from build123d import *

# Parameters (mm, degrees)
SKETCH_1_W      = 40
SKETCH_1_H      = 40
EXTRUDE_1_DEPTH = 20
CHAMFER_2_SIZE  = 2
SKETCH_2_R      = 5
EXTRUDE_3_DEPTH = 2
SKETCH_4_R      = 2.5
EXTRUDE_6_DEPTH = 3
CHAMFER_3_SIZE  = 2
FILLET_1_R      = 2


with BuildPart() as part:
    # 草图1 → 凸台-拉伸1 (new body)
    with BuildSketch(Plane.XY):
        with Locations((-8.736097926, 20.42824298)):
            Rectangle(SKETCH_1_W, SKETCH_1_H)
    extrude(amount=EXTRUDE_1_DEPTH)

    # 倒角2
    chamfer_2_edges = [part.edges().sort_by_distance(p)[0] for p in [
        (-8.736097926, 40.42824298, 20),
        (-8.736097926, 40.42824298, 0),
        (-28.736097926, 40.42824298, 10),
        (11.263902074, 40.42824298, 10),
    ]]
    chamfer(chamfer_2_edges, length=CHAMFER_2_SIZE)

    # 草图2 → 凸台-拉伸3 (add)
    with BuildSketch(Plane(origin=(0, 0.42824298, 0), x_dir=(-1, 0, 0), z_dir=(0, -1, 0))):
        with Locations(Location((18.736097926, -10, 0), (0, 0, 270))):
            Circle(SKETCH_2_R)
    extrude(amount=EXTRUDE_3_DEPTH)

    # 草图4 → 凸台-拉伸6 (add)
    with BuildSketch(Plane.XZ.offset(1.57175702)):
        with Locations(Location((-18.736097926, 10, 0), (0, 0, 270))):
            Circle(SKETCH_4_R)
    extrude(amount=EXTRUDE_6_DEPTH)

    # 倒角3
    chamfer_3_edges = [part.edges().sort_by_distance(p)[0] for p in [
        (-8.736097926, 0.42824298, 20),
        (-8.736097926, 0.42824298, 0),
        (-28.736097926, 0.42824298, 10),
        (11.263902074, 0.42824298, 10),
    ]]
    chamfer(chamfer_3_edges, length=CHAMFER_3_SIZE)

    # 圆角1
    fillet_1_edges = [part.edges().sort_by_distance(p)[0] for p in [
        (11.263902074, 20.42824298, 0),
        (11.263902074, 20.42824298, 20),
        (-28.736097926, 20.42824298, 0),
        (-28.736097926, 20.42824298, 20),
    ]]
    fillet(fillet_1_edges, radius=FILLET_1_R)


solid = part.part
Model file for the job. Use its own axes, mm. A direction names the side the tool comes from. Round coordinates to 2 decimals unless told otherwise and drop trailing zeros. Loops run counter-clockwise (first coordinate to the right, second up) from the corner with the lowest first, then second, coordinate; pieces in that order, holes last. Notation, with made-up numbers: (67.25, -27.5) - (93.25, -27.5) arc R16 ccw to (93.25, -17.5) - close; hole circle Ø9 at (38, 83). An arc over 180 degrees is marked (long way). Write each question's results on one line, items separated by ' | '.
(1) Saw through at D-D, the plane x = -18. List the corners of the cut face in (y, z), then the cut area to 3 significant figures.
Answer below:
outline: (-4.57, 7.61) - (-1.57, 7.61) - (-1.57, 5.05) - (0.43, 5.05) - (0.43, 2) - (2.43, 0) - (38.43, 0) - (40.43, 2) - (40.43, 18) - (38.43, 20) - (2.43, 20) - (0.43, 18) - (0.43, 14.95) - (-1.57, 14.95) - (-1.57, 12.39) - (-4.57, 12.39) - close | area: 826 mm^2
(2) Pin check, flat tips, straight feed: pin 1 (6 mm diameter, centred on x = 7, z = 12, fed in from -Y); pin 2 (3 mm diameter, centred on x = -14, z = 7, fed in from -Y). Stop position of each tip, or through.
Answer below:
pin 1: stops at y = 0.43 | pin 2: stops at y = -1.57
(3) Wall check: L1, parallel to Y at x = -23, z = 3.5; L2, parallel to Y at x = -23, z = 9.5; L3, parallel to Z at x = -16.5, y = 0. Give the ranges that are in metal, low to high.
Answer below:
L1: y = 0.43 to 40.43 | L2: y = -1.57 to 40.43 | L3: z = 5.53 to 14.47
(4) Saw through at A-A, the plane x = -11.5. List the corners of the cut face in (y, z), then the cut area to 3 significant figures.
Answer below:
outline: (0.43, 2) - (2.43, 0) - (38.43, 0) - (40.43, 2) - (40.43, 18) - (38.43, 20) - (2.43, 20) - (0.43, 18) - close | area: 792 mm^2
(5) Saw through at C-C, the plane z = 6. List the corners of the cut face in (x, y), then the cut area to 3 significant figures.
Answer below:
outline: (-28.74, 2.43) - (-26.74, 0.43) - (-21.74, 0.43) - (-21.74, -1.57) - (-15.74, -1.57) - (-15.74, 0.43) - (9.26, 0.43) - (11.26, 2.43) - (11.26, 38.43) - (9.26, 40.43) - (-26.74, 40.43) - (-28.74, 38.43) - close | area: 1,600 mm^2
(6) 3-axis set-ups, long thin cutter, end or side, ignore diameter. For faces 1 (the flat face through (-16.6, -1.572, 12.2)), 2 (the flat face through (-27.72, 1.41, 9.87)): which of +Z, -Z, +X, -X, +Y, -Y reach the whole face in a straight line?
Answer below:
face 1: -Y | face 2: +Z, -Z, -X, -Y
(7) Saw through at B-B, the plane z = 10. List the corners of the cut face in (x, y), then the cut area to 3 significant figures.
Answer below:
outline: (-28.74, 2.43) - (-26.74, 0.43) - (-23.74, 0.43) - (-23.74, -1.57) - (-21.24, -1.57) - (-21.24, -4.57) - (-16.24, -4.57) - (-16.24, -1.57) - (-13.74, -1.57) - (-13.74, 0.43) - (9.26, 0.43) - (11.26, 2.43) - (11.26, 38.43) - (9.26, 40.43) - (-26.74, 40.43) - (-28.74, 38.43) - close | area: 1,630 mm^2
